Check sheet for the modelled part. Datum: model origin and axes. Units: mm. A direction names the side the tool comes from. Round coordinates to 2 decimals unless told otherwise and drop trailing zeros. Order: outer loops, then holes, each group sorted by start corner. A loop starts at its lowest first (then second) coordinate and runs counter-clockwise, first axis right, second up. Notation, with made-up numbers: (-38.75, 4.25) -> (-9.75, 4.25) arc R22 cw to (-9.75, 28.25) -> close; hole circle Ø5 at (3, -12). An arc over 180 degrees is marked (long way). Answer in a Markdown table with one row per item.
Autodesk Inventor part; units mm, degrees
ref_plane "YZ Plane" through (0, 0, 0) normal (1, 0, 0) x (0, 1, 0)
ref_plane "XZ Plane" through (0, 0, 0) normal (0, 1, 0) x (-1, 0, 0)
ref_plane "XY Plane" through (0, 0, 0) normal (0, 0, 1) x (1, 0, 0)
sketch "Sketch1" plane through (0, 0, 0) normal (0, 1, 0) x (-1, 0, 0)
  circle A0 centre (0, 0) radius 2
  line L0 (-7.4162, 0) -> (-12.5838, 0) construction
  circle A1 centre (-20, 0) radius 2
  arc A2 (-4.6351, -1.875) -> (0, 5) centre (0, 0) ccw
  arc A3 (-24.6351, -1.875) -> (-15.3649, -1.875) centre (-20, 0) ccw
  line L1 (-5, 0) -> (-15, 0)
  arc A4 (-4.6351, -1.875) -> (-7.4162, 0) centre (-7.4162, -3) ccw
  arc A5 (-12.5838, 0) -> (-15.3649, -1.875) centre (-12.5838, -3) ccw
  line L2 (-27.4162, 0) -> (-74.7698, 0) construction
  line L3 (-80, 0) -> (-80, 12.5) construction
  line L4 (-80, 12.5) -> (-60, 12.5) construction
  line L5 (-75.5648, 2.772) -> (-62.295, 11.0656)
  line L6 (-80, 0) -> (-25, 0)
  line L7 (0, 5) -> (-57, 5)
  line L8 (-60, 8) -> (-60, 9.7936)
  arc A6 (-60, 8) -> (-57, 5) centre (-57, 8) ccw
  arc A7 (-60, 9.7936) -> (-62.295, 11.0656) centre (-61.5, 9.7936) ccw
  arc A8 (-75.5648, 2.772) -> (-74.7698, 0) centre (-74.7698, 1.5) ccw
  arc A9 (-24.6351, -1.875) -> (-27.4162, 0) centre (-27.4162, -3) ccw
  point P0 (-60, 5)
  point P1 (0, 5)
  point P2 (-74.7698, 0)
  point P3 (-7.4162, 0)
  point P4 (-27.4162, 0)
  dimension "d0" = 4
  dimension "d4" = 4
  dimension "d5" = 10
  dimension "d6" = 10
  dimension "d7" = 3
  dimension "d8" = 80
  dimension "d9" = 12.5
  dimension "d10" = 20
  dimension "d11" = 60
  dimension "d12" = 3
  dimension "d13" = 1.5
  dimension "d19" = 5
  dimension "d20" = 3
extrude "Extrusion1" add sketch "Sketch1" along normal blind 10
chamfer "Chamfer1" distance 0.25 angle 45 4 edges at (22, 10, 0) (2, 10, 0) (22, 0, 0) (2, 0, 0)
sketch "Sketch2" plane through (0, 10, 0) normal (0, 1, 0) x (1, 0, 0)
  circle A0 centre (20, 0) radius 2.25
  arc A1 (75.5648, -2.772) -> (74.7698, 0) centre (74.7698, -1.5) ccw
  line L0 (74.7698, 0) -> (27.4162, 0)
  arc A2 (24.6351, 1.875) -> (27.4162, 0) centre (27.4162, 3) ccw
  arc A3 (24.6351, 1.875) -> (15.3649, 1.875) centre (20, 0) ccw
  arc A4 (12.5838, 0) -> (15.3649, 1.875) centre (12.5838, 3) ccw
  line L1 (12.5838, 0) -> (7.4162, 0)
  arc A5 (4.6351, 1.875) -> (7.4162, 0) centre (7.4162, 3) ccw
  arc A6 (4.6351, 1.875) -> (0, -5) centre (0, 0) ccw
  line L2 (0, -5) -> (57, -5)
  arc A7 (60, -8) -> (57, -5) centre (57, -8) ccw
  line L3 (60, -8) -> (60, -9.7936)
  arc A8 (60, -9.7936) -> (62.295, -11.0656) centre (61.5, -9.7936) ccw
  line L4 (62.295, -11.0656) -> (75.5648, -2.772)
  circle A9 centre (0, 0) radius 2.25
sketch "Sketch3" plane through (0, 10, 0) normal (0, 1, 0) x (1, 0, 0)
  line L0 (27.4162, 0) -> (27.4162, -5) construction
  line L1 (0, -5) -> (57, -5) construction
  line L2 (27.4162, 0) -> (30.4162, 0) construction
  line L3 (30.4162, 0) -> (30.4162, -5) construction
  line L4 (30.4162, -5) -> (27.4162, -5) construction
  line L5 (27.4162, -5) -> (27.4162, 0) construction
  line L6 (30.4162, 0) -> (45.4162, 0) construction
  line L7 (74.7698, 0) -> (27.4162, 0)
  line L8 (30.4162, -1.25) -> (45.4162, -1.25)
  line L9 (45.4162, 1.25) -> (30.4162, 1.25)
  arc A0 (30.4162, 1.25) -> (30.4162, -1.25) centre (30.4162, 0) ccw
  arc A1 (45.4162, -1.25) -> (45.4162, 1.25) centre (45.4162, 0) ccw
  line L10 (30.4162, -5) -> (45.4162, -5) construction
  line L11 (30.4162, -6.25) -> (45.4162, -6.25)
  line L12 (45.4162, -3.75) -> (30.4162, -3.75)
  arc A2 (30.4162, -3.75) -> (30.4162, -6.25) centre (30.4162, -5) ccw
  arc A3 (45.4162, -6.25) -> (45.4162, -3.75) centre (45.4162, -5) ccw
  point P0 (0, 0)
  point P1 (37.9162, 0)
  point P2 (37.9162, -5)
  point P3 (46.6662, 0)
  point P4 (29.1662, 0)
  dimension "d21" = 3
  dimension "d22" = 5
  dimension "d28" = 15
  dimension "d29" = 2.5
  dimension "d30" = 15
  dimension "d31" = 2.5
extrude "Extrusion2" cut sketch "Sketch3" against normal through all contours A1 L8 A0 L7 | A2 L12 A3 L11
fillet "Fillet2" radius 5 4 edges at (29.1662, 5, 0) (46.6662, 5, 0) (46.6662, 5, 5) (29.1662, 5, 5)
properties part number "Battery_Clip" material "Nylon 6/6"
(1) Section check B-B on y = 6. Give the number of separate pieces and of enclosed holes in the cut face, plus the area to 3 significant figures.
Solutions:
| item | result |
|---|---|
| separate pieces | 1 |
| enclosed holes | 2 |
| area | 452 mm^2 |
(2) Draft check along Z on faces 1 (the cylindrical face through (21.6, 4.9, 1.2)), 2 (the cylindrical face through (25.63, 4.93, -0.59)), 3 (the cylindrical face through (28.23, 5.07, 4.75)). Enter one of: pulls with the +Z half, pulls with the -Z half, needs draft (parallel to the pull), parting line crosses it, or undercut.
Solutions:
| item | result |
|---|---|
| face 1 | undercut |
| face 2 | pulls with the -Z half |
| face 3 | pulls with the +Z half |
(3) Section check D-D on z = 7. Record the boundary of the cut face in (x, y).
Solutions:
| item | result |
|---|---|
| outline | (59.83, 0) -> (68.8, 0) -> (68.8, 10) -> (59.83, 10) -> close |
(4) Section check C-C on x = 35. Record the boundary of the cut face in (y, z).
Solutions:
| item | result |
|---|---|
| outline | (0, 1.25) -> (10, 1.25) -> (10, 3.75) -> (0, 3.75) -> close |
(5) Depth check by flat-ended pin: pin 1 Ø1 at (x, y) = (59.5, 5.5) entering from -Z; pin 2 Ø4 at (x, y) = (35, 8) entering from +Z; pin 3 Ø5 at (x, y) = (12, 7.5) entering from +Z. Enter the tip coordinate at first touch or a pass-through.
Solutions:
| item | result |
|---|---|
| pin 1 | z = 0 |
| pin 2 | z = 3.75 |
| pin 3 | z = 5 |
(6) Tool access check on faces 4 (the flat face through (69.023, 4.93, 6.861)), 5 (the cylindrical face through (14.281, 4.93, -0.527)), 6 (the flat face through (53, 5, 5)), 7 (the cylindrical face through (47.564, 5.07, 4.736)). Record the directions out of +Z, -Z, +X, -X, +Y, -Y that give a thin tool (end or side, any length) a straight path to the whole face; none if there is none.
Solutions:
| item | result |
|---|---|
| face 4 | +Z, +X, +Y, -Y |
| face 5 | -Z, +Y, -Y |
| face 6 | +Z, -X, +Y, -Y |
| face 7 | +Z, +Y, -Y |
(7) Section check A-A on x = 20. Record the boundary of the cut face in (y, z), plus the area to 3 significant figures.
Solutions:
| item | result |
|---|---|
| outline | (0, -5) -> (10, -5) -> (10, -2.25) -> (9.75, -2) -> (0.25, -2) -> (0, -2.25) -> close; (0, 2.25) -> (0.25, 2) -> (9.75, 2) -> (10, 2.25) -> (10, 5) -> (0, 5) -> close |
| area | 59.9 mm^2 |
(8) Scan lines: probe 1 along Z at (x, y) = (0, 7.25); probe 2 along Z at (x, y) = (7, 9); probe 3 along X at (y, z) = (9.75, 4). Record each from-to range of solid material in increasing order. Write a range as from..to.
Solutions:
| item | result |
|---|---|
| probe 1 | -5..-2, 2..5 |
| probe 2 | -0.03..5 |
| probe 3 | -3..29.67, 46.17..73.6 |
